Input: part model. Units: mm. Frame: model coordinates. A direction names the side the tool comes from. Coordinates: 2 decimals unless noted, no trailing zeros. Loops run counter-clockwise (first coordinate to the right, second up) from the corner with the lowest first, then second, coordinate; pieces in that order, holes last. Notation, with made-up numbers: (-6.75, 8) -> (50.25, 8) arc R7 ccw to (50.25, 18) -> close; hole circle Ø3 at (54, -23.75). An arc over 180 degrees is marked (long way). Put each result on its own line as item: value. Start each with the question number.
1) Cut plane B-B (x = -49). Return the cut outline in (y, z).
2) Cut plane A-A (y = 2). Return the cut outline in (x, z), plus the area to 3 significant figures.
3) Pull-direction query (Y, two-part tool) for faces 5 (the flat face through (-50, 21.635, 76)), 6 (the flat face through (-36.035, 10, 60)), 7 (the flat face through (-38, -42.365, 60)), 8 (the flat face through (-50, 14, 72)); classes: pulls with the +Y half, pulls with the -Y half, needs draft (parallel to the pull), parting line crosses it, or undercut.
4) Material intervals for L1, parallel to Z at x = 7.5, y = 10; L2, parallel to X at y = 22, z = 75; L3, parallel to Z at x = -53, y = -20, sorted ascending.
5) Cut plane D-D (y = -35). Return the cut outline in (x, z), plus the area to 3 significant figures.
6) Cut plane C-C (z = 70). Return the cut outline in (x, y).
7) Set-up query: faces 1 (the flat face through (4, 5, 24)), 2 (the flat face through (-50, 5.635, 76)), 3 (the flat face through (-4, 21.635, 12)), 4 (the flat face through (-12.035, -17, 16)). Return all of +Z, -Z, +X, -X, +Y, -Y with unobstructed straight access to the full face (end or side cutting, diameter ignored); none if empty.
8) Contact query for flat-ended pins moving along their axis: P1, Ø8, axis at x = -7, z = 16, coming from the +Y side; P2, Ø9.5, axis at x = 7.5, z = 41, coming from the +Y side; P3, Ø10, axis at y = -20.5, z = 46, coming from the +X side. Output: stop coordinate, or through.
from build123d import *

# Parameters (mm, degrees)
BOSS_EXTRUDE1_DEPTH = 80
SKETCH2_W           = 56
SKETCH2_H           = 40
CUT_EXTRUDE1_DEPTH  = 32
SKETCH3_W           = 52
SKETCH3_H           = 40
CUT_EXTRUDE2_DEPTH  = 100
CUT_EXTRUDE3_DEPTH  = 100
SKETCH5_W           = 8
SKETCH5_H           = 16
CUT_EXTRUDE4_DEPTH  = 100


with BuildPart() as part:
    # Sketch1 → Boss-Extrude1 (new body)
    with BuildSketch(Plane.XY):
        with BuildLine():
            Line((-64.034777708, 29.634699451), (-36.034777708, 29.634699451))
            Line((-36.034777708, 29.634699451), (-36.034777708, -10.365300549))
            ThreePointArc((-36.034777708, -10.365300549), (-24.034777708, -22.365300549), (-12.034777708, -10.365300549))
            Line((-12.034777708, -10.365300549), (-12.034777708, 21.634699451))
            Line((-12.034777708, 21.634699451), (3.965222292, 21.634699451))
            ThreePointArc((3.965222292, 21.634699451), (15.278930791, 16.94840795), (19.965222292, 5.634699451))
            Line((19.965222292, 5.634699451), (19.965222292, -10.365300549))
            ThreePointArc((19.965222292, -10.365300549), (10.59263929, -32.992717547), (-12.034777708, -42.365300549))
            Line((-12.034777708, -42.365300549), (-64.034777708, -42.365300549))
            Line((-64.034777708, -42.365300549), (-64.034777708, 29.634699451))
        make_face()
    extrude(amount=BOSS_EXTRUDE1_DEPTH)

    # Sketch2 → Cut-Extrude1 (cut)
    with BuildSketch(Plane(origin=(19.965222292, 0, 0), x_dir=(0, 0, -1), z_dir=(1, 0, 0))):
        with Locations((-52, 9.634699451)):
            Rectangle(SKETCH2_W, SKETCH2_H)
    extrude(amount=-CUT_EXTRUDE1_DEPTH, mode=Mode.SUBTRACT)

    # Sketch3 → Cut-Extrude2 (cut)
    with BuildSketch(Plane(origin=(0, 29.634699451, 0), x_dir=(1, 0, 0), z_dir=(0, 1, 0))):
        with Locations((-38.034777708, -20)):
            Rectangle(SKETCH3_W, SKETCH3_H)
    extrude(amount=-CUT_EXTRUDE2_DEPTH, mode=Mode.SUBTRACT)

    # Sketch4 → Cut-Extrude3 (cut)
    with BuildSketch(Plane(origin=(-36.034777708, 0, 0), x_dir=(0, 0, -1), z_dir=(1, 0, 0))):
        Polygon((-40, 29.634699451), (-40, 5.634699451), (-52, 29.634699451), align=None)
    extrude(amount=-CUT_EXTRUDE3_DEPTH, mode=Mode.SUBTRACT)

    # Sketch5 → Cut-Extrude4 (cut)
    with BuildSketch(Plane(origin=(0, 0, 0), x_dir=(0, 0, -1), z_dir=(1, 0, 0))):
        with Locations((-76, 13.634699451)):
            Rectangle(SKETCH5_W, SKETCH5_H)
    extrude(amount=-CUT_EXTRUDE4_DEPTH, mode=Mode.SUBTRACT)


solid = part.part
Results found:
1. outline: (-42.37, 40) -> (5.63, 40) -> (29.63, 52) -> (29.63, 80) -> (21.63, 80) -> (21.63, 72) -> (5.63, 72) -> (5.63, 80) -> (-42.37, 80) -> close
2. outline: (-64.03, 40) -> (-36.03, 40) -> (-36.03, 80) -> (-64.03, 80) -> close; (-12.03, 0) -> (19.97, 0) -> (19.97, 24) -> (-12.03, 24) -> close
2. area: 1,890 mm2
3. face 5: undercut
3. face 6: needs draft
3. face 7: pulls with the -Y half
3. face 8: undercut
4. L1: z = 0 to 24
4. L2: x = -64.03 to -36.03
4. L3: z = 40 to 80
5. outline: (-64.03, 40) -> (-12.03, 40) -> (-12.03, 0) -> (8.39, 0) -> (8.39, 80) -> (-64.03, 80) -> close
5. area: 3,710 mm2
6. outline: (-64.03, -42.37) -> (-12.03, -42.37) arc R32 ccw to (19.97, -10.37) -> (-12.03, -10.37) arc R12 cw to (-36.03, -10.37) -> (-36.03, 29.63) -> (-64.03, 29.63) -> close
7. face 1: +Z, +X, -X, +Y
7. face 2: +Z, +X, -X
7. face 3: +Z, -Z, +X, -X, +Y
7. face 4: -Z, -X, +Y, -Y
8. P1: stops at y = 21.63
8. P2: stops at y = -10.37
8. P3: stops at x = 19.55
